Autodesk Inventor part; units mm, degrees
ref_plane "YZ Plane" through (0, 0, 0) normal (1, 0, 0) x (0, 1, 0)
ref_plane "XZ Plane" through (0, 0, 0) normal (0, 1, 0) x (-1, 0, 0)
ref_plane "XY Plane" through (0, 0, 0) normal (0, 0, 1) x (1, 0, 0)
sketch "Sketch1" plane through (0, 0, 0) normal (0, 1, 0) x (-1, 0, 0)
  line L0 (0, 0) -> (30, 0)
  line L1 (30, 0) -> (30, -30)
  line L2 (30, -30) -> (0, -30)
  line L3 (0, -30) -> (0, 0)
  dimension "d0" = 30
  dimension "d1" = 30
extrude "Extrusion1" add sketch "Sketch1" along normal blind 30
sketch "Sketch2" plane through (0, 30, 0) normal (0, 1, 0) x (1, 0, 0)
  line L0 (-20, 17.25) -> (-10, 17.25)
  line L1 (-10, 17.25) -> (-10, 12.75)
  line L2 (-10, 12.75) -> (-20, 12.75)
  line L3 (-20, 12.75) -> (-20, 17.25)
  line L4 (-20, 17.25) -> (-10, 12.75) construction
  line L5 (-10, 17.25) -> (-20, 12.75) construction
  line L6 (-30, 30) -> (-30, 0)
  line L7 (-30, 0) -> (0, 0)
  point P0 (-15, 15)
  point P1 (-30, 15)
  dimension "d4" = 15
  dimension "d5" = 15
  dimension "d6" = 10
  dimension "d7" = 4.5
extrude "Extrusion2" add sketch "Sketch2" along normal blind 20
sketch "Sketch3" plane through (-20, 30, -12.75) normal (0, 0, 1) x (1, 0, 0)
  circle A0 centre (5, 14.8617) radius 2.6
  point P0 (20, -30)
  dimension "d10" = 5.2
extrude "Extrusion3" cut sketch "Sketch3" against normal blind 20
sketch "Sketch4" plane through (-30, 0, 0) normal (0, 0, 1) x (1, 0, 0)
  circle A0 centre (15, 15) radius 15
  line L0 (0, 30) -> (30, 30)
  line L1 (0, 0) -> (30, 0)
  line L2 (30, 0) -> (30, 30)
  line L3 (30, 30) -> (0, 30)
  line L4 (0, 30) -> (0, 0)
  line L5 (0, 0) -> (30, 30) construction
  line L6 (30, 0) -> (0, 30) construction
  point P0 (0, 15)
  point P1 (15, 30)
  point P2 (30, 15)
  point P3 (15, 0)
  dimension "d13" = 15
  dimension "d14" = 30
extrude "Extrusion4" cut sketch "Sketch4" against normal blind 71.25 contours L2 L1 A0 | A0 L0 L2 | A0 L4 L0 | L1 L4 A0
sketch "Sketch5" plane through (-15, 30, -17.25) normal (0, -1, 0) x (1, 0, 0)
  line L0 (-5.2786, 4.8714) -> (5, 4.8714)
  line L1 (5, 4.8714) -> (5, 0)
  line L2 (5, 0) -> (-5.2786, 0)
  line L3 (-5.2786, 0) -> (-5.2786, 4.8714)
  point P0 (15, 17.25)
extrude "Extrusion5" add sketch "Sketch5" along normal blind 5
properties part number "ObjectCylinder"
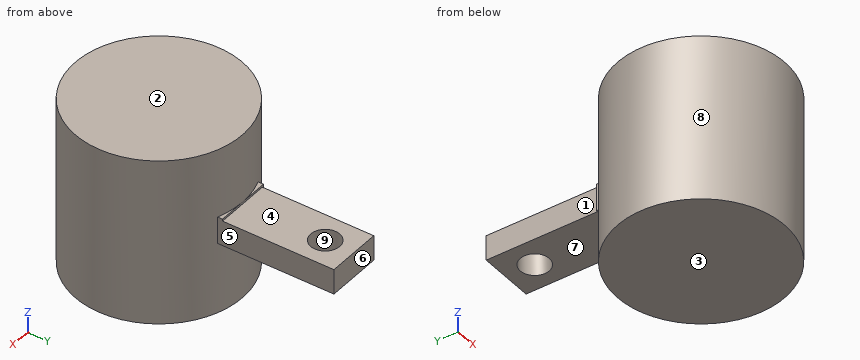
Geometry: final body of the model. Coordinates: model frame, mm. Face numbers are marked on the shaded views. A direction names the side the tool comes from. Coordinates: 2 decimals unless noted, no trailing zeros. Order: outer loops, then holes, each group sorted by start corner. A loop starts at its lowest first (then second) coordinate and runs counter-clockwise, first axis right, second up.
(1) Material intervals for probe 1 along Y at (x, z) = (-15, -15.7); probe 2 along Z at (x, y) = (-14, 41); probe 3 along X at (y, z) = (26, -22.5), sorted ascending.
(2) Access query for the marked faces 1, 2, 3, 4 and 5. Directions: +Z, -Z, +X, -X, +Y, -Y. A direction counts if a zero-diameter tool reaches every point of the face in a straight line with its end or side. Return the directions, or none.
(3) Section query B-B (y = 36.5). Return the cut outline in (x, z).
(4) First-contact query: pin 1 (3.5 mm diameter, centred on y = 41, z = -15.5, fed in from -X); pin 2 (2 mm diameter, centred on y = 29.5, z = -15, fed in from -X); pin 3 (8 mm diameter, centred on x = -19.5, z = -7.5, fed in from +Y). Flat tips, straight axial feed; report the tip coordinate or a pass-through.
(5) Draft query along Y for the marked faces 6, 7, 8 and 9. Return one class per face: pulls with the +Y half, pulls with the -Y half, needs draft (parallel to the pull), parting line crosses it, or undercut.
(6) Section query A-A (z = -13.5). Return the cut outline in (x, y).
(7) Section query C-C (x = -8.5). Return the cut outline in (y, z).
Solution:
1. probe 1: y = 0 to 42.26, 47.46 to 50
1. probe 2: z = -17.25 to -12.75
1. probe 3: x = -25.2 to -4.8
2. face 1: +Z, -Z, -X, +Y
2. face 2: +Z, +X, -X, +Y, -Y
2. face 3: -Z, +X, -X, +Y, -Y
2. face 4: +Z, +X, -X, +Y
2. face 5: +Z, -Z, +X, +Y
3. outline: (-20, -17.25) - (-10, -17.25) - (-10, -12.75) - (-20, -12.75) - close
4. pin 1: stops at x = -20
4. pin 2: stops at x = -21.54
4. pin 3: stops at y = 29.99
5. face 6: pulls with the +Y half
5. face 7: needs draft
5. face 8: parting line crosses it
5. face 9: undercut
6. outline: (-20.28, 29.04) arc R15 ccw (long way) to (-10, 29.14) - (-10, 50) - (-20, 50) - (-20, 30) - (-20.28, 30) - close; hole circle Ø5.2 at (-15, 44.86)
7. outline: (1.48, -30) - (28.52, -30) - (28.52, 0) - (1.48, 0) - close
